Autodesk Inventor part; units mm, degrees
ref_plane "YZ Plane" through (0, 0, 0) normal (1, 0, 0) x (0, 1, 0)
ref_plane "XZ Plane" through (0, 0, 0) normal (0, 1, 0) x (-1, 0, 0)
ref_plane "XY Plane" through (0, 0, 0) normal (0, 0, 1) x (1, 0, 0)
sketch "Sketch1" plane through (0, 0, 0) normal (0, 0, 1) x (1, 0, 0)
  line L0 (0, 0) -> (15, 0)
  line L1 (15, 0) -> (15, 27)
  line L2 (15, 27) -> (0, 27)
  line L3 (0, 27) -> (0, 0)
  circle A0 centre (7.5, 30) radius 4
  circle A1 centre (7.5, 30) radius 1.5
  point P0 (7.5, 27)
  dimension "d2" = 15
  dimension "d3" = 27
  dimension "d7" = 8
  dimension "d8" = 3
  dimension "d9" = 3
extrude "Extrusion1" add sketch "Sketch1" along normal blind 15
sketch "Sketch2" plane through (0, 0, 15) normal (0, 0, 1) x (1, 0, 0)
  circle A0 centre (7.5, 30) radius 1.5
  line L0 (0, 27) -> (0, 0)
  line L1 (0, 0) -> (15, 0)
  line L2 (15, 0) -> (15, 27)
  circle A1 centre (7.5, 30) radius 4
  arc A2 (10.1458, 27) -> (4.8542, 27) centre (7.5, 30) ccw
  line L3 (4.25, 3) -> (10.75, 3)
  line L4 (10.75, 3) -> (10.75, 24)
  line L5 (10.75, 24) -> (4.25, 24)
  line L6 (4.25, 24) -> (4.25, 3)
  point P0 (11.4441, 29.3333)
  point P1 (3.5559, 29.3333)
  point P2 (10.75, 13.5)
  point P3 (15, 13.5)
  point P4 (7.5, 3)
  point P5 (7.5, 0)
  dimension "d14" = 6.5
  dimension "d16" = 21
extrude "Extrusion2" cut sketch "Sketch2" against normal blind 10
fillet "Fillet2" radius 3 2 edges at (10.1458, 27, 2.5) (4.8542, 27, 2.5)
sketch "Sketch3" plane through (0, 0, 5) normal (0, 0, 1) x (1, 0, 0)
  line L0 (10.75, 3) -> (4.25, 3) construction
  line L1 (10.75, 24) -> (10.75, 3) construction
  line L2 (4.25, 24) -> (10.75, 24) construction
  line L3 (4.25, 3) -> (4.25, 24) construction
  line L4 (5.25, 23) -> (9.75, 23)
  line L5 (9.75, 23) -> (9.75, 4)
  line L6 (9.75, 4) -> (5.25, 4)
  line L7 (5.25, 4) -> (5.25, 23)
  point P0 (0, 0)
  dimension "d20" = 1
extrude "Extrusion3" cut sketch "Sketch3" against normal blind 10
properties part number "relay1"
CAD build for the part. Positions are in the model's coordinates, mm. A direction names the side the tool comes from. Round coordinates to 2 decimals unless told otherwise and drop trailing zeros. Loops run counter-clockwise (first coordinate to the right, second up) from the corner with the lowest first, then second, coordinate; pieces in that order, holes last. Notation, with made-up numbers: M 41,69 L 53,69 A17 cw 53,94 Z; hole C 17,42 d5. An arc over 180 degrees is marked long. Return JSON: item names as keys, results as strings. Group by question number.
(1) Drop flat-ended pins along their axis: P1, Ø5, axis at x = 8, y = 18, coming from the +Z side; P2, Ø1.5, axis at x = 2.5, z = 4.5, coming from the +Y side; P3, Ø5, axis at x = 3, z = 8, coming from the +Y side. Give the stop position or say it passes through.
(2) Saw through at C-C, the plane y = 19.5. List the corners of the cut face in (x, z), and give its area (4 significant figures).
(3) Saw through at A-A, the plane x = 7.5. List the corners of the cut face in (y, z), and give its area (3 significant figures).
(4) Saw through at D-D, the plane z = 2.5. List the corners of the cut face in (x, y).
(5) Tool access for faces 1 (the flat face through (8, 24, 10)), 2 (the flat face through (7, 23, 3)), 3 (the cylindrical face through (7.5, 26, 10.1)): list every direction of +Z, -Z, +X, -X, +Y, -Y with a clear straight run to the whole face (end or side of a thin tool).
(6) Wall check: probe 1 along Y at (x, z) = (7.5, 3.3); probe 2 along X at (y, z) = (10, 11); probe 3 along X at (y, z) = (17.5, 4.5). Give the ranges that are in metal, low to high. Write a range as [from, to].
(7) Mould opens along X. For faces 4 (the cylindrical face through (2.6, 27.86, 2.54)), 5 (the flat face through (9.75, 14, 3)), 6 (the flat face through (8, 4, 3)), 7 (the flat face through (15, 13, 7)) say: +X half, -X half, draft (parallel to the pull), parting line (faces both ways), or undercut.
(8) Saw through at B-B, the plane z = 6.25. List the corners of the cut face in (x, y), and give its area (3 significant figures).
Answer list:
{
 "1": {"P1": "z = 5", "P2": "y = 28.8", "P3": "y = 27"},
 "2": {"outline": "M 0,0 L 5.25,0 L 5.25,5 L 4.25,5 L 4.25,15 L 0,15 Z; M 9.75,0 L 15,0 L 15,15 L 10.75,15 L 10.75,5 L 9.75,5 Z", "area": "137.5 mm2"},
 "3": {"outline": "M 0,0 L 4,0 L 4,5 L 3,5 L 3,15 L 0,15 Z; M 23,0 L 28.5,0 L 28.5,5 L 26,5 L 26,15 L 24,15 L 24,5 L 23,5 Z; M 31.5,0 L 34,0 L 34,5 L 31.5,5 Z", "area": "110 mm2"},
 "4": {"outline": "M 0,0 L 15,0 L 15,27 L 14.5,27 A3 cw 11.5,30 A4 ccw 3.5,30 A3 cw 0.5,27 L 0,27 Z; hole M 5.25,4 L 9.75,4 L 9.75,23 L 5.25,23 Z; hole C 7.5,30 d3"},
 "5": {"face 1": "+Z", "face 2": "+Z, -Z", "face 3": "+Z, +Y"},
 "6": {"probe 1": "[0, 4], [23, 28.5], [31.5, 34]", "probe 2": "[0, 4.25], [10.75, 15]", "probe 3": "[0, 5.25], [9.75, 15]"},
 "7": {"face 4": "-X half", "face 5": "undercut", "face 6": "undercut", "face 7": "+X half"},
 "8": {"outline": "M 0,0 L 15,0 L 15,27 L 10.15,27 A4 cw 4.85,27 L 0,27 Z; hole M 4.25,3 L 10.75,3 L 10.75,24 L 4.25,24 Z", "area": "265 mm2"}
}
